Check sheet for the modelled part. Datum: model origin and axes. Units: mm. Round coordinates to 2 decimals unless told otherwise and drop trailing zeros. Loops run counter-clockwise (first coordinate to the right, second up) from the corner with the lowest first, then second, coordinate; pieces in that order, holes last. Notation, with made-up numbers: (48, 37.25) - (69, 37.25) arc R18 ccw to (69, 44.25) - close; hole circle Ø9 at (85, 34.25). An arc over 180 degrees is marked (long way). Put each result on its own line as item: value. Start each with the question number.
Item 1: Section check B-B, the plane x = 1.5. Record the cut outline in (y, z), and give its area (3 significant figures).
Item 2: Gauge pin test, flat ends, axial feed: pin 1 Ø4 at (x, y) = (5.5, -7.5) entering from -Z; pin 2 Ø2 at (x, z) = (3.5, -6) entering from +Y; pin 3 Ø6 at (x, z) = (7, -2) entering from -Y. Record the tip position at first contact, or that the pin passes through.
Item 3: Section check A-A, the plane y = 0. Record the cut outline in (x, z) (3 decimals).
Item 4: Draft check along Z on faces 1 (the flat face through (5.33, 7.76, 4.56)), 2 (the flat face through (5.33, 7.83, -4.44)), 3 (the cylindrical face through (5.33, -3.51, 3.82)), 4 (the flat face through (0, 2, -6)). Enter one of: pulls with the +Z half, pulls with the -Z half, needs draft (parallel to the pull), parting line crosses it, or undercut.
Item 5: Material ranges on line 1 along Z through (x, y) = (6.25, 0); line 2 along Z through (x, y) = (9.25, 3.75); line 3 along Y through (x, z) = (2, -1.75), recorded low to high.
Autodesk Inventor part; units mm, degrees
ref_plane "Work Plane1" through (-18.9656, 0, 0) normal (0, -0.8660254, -0.5) x (1, 0, 0)
ref_plane "YZ Plane" through (0, 0, 0) normal (1, 0, 0) x (0, 1, 0)
ref_plane "XZ Plane" through (0, 0, 0) normal (0, 1, 0) x (-1, 0, 0)
sketch "Эскиз1" plane through (0, 0, 0) normal (1, 0, 0) x (0, 1, 0)
  line L0 (-10.3923, 0) -> (-5.1962, 9)
  line L1 (-5.1962, 9) -> (5.1962, 9)
  line L2 (5.1962, 9) -> (10.3923, 0)
  line L3 (10.3923, 0) -> (5.1962, -9)
  line L4 (5.1962, -9) -> (-5.1962, -9)
  line L5 (-5.1962, -9) -> (-10.3923, 0)
  point P0 (0, 0)
  point P1 (0, 0)
  dimension "d0" = 20.7846
extrude "Базовый элемент" add sketch "Эскиз1" along normal blind 10.8
sketch "Эскиз2" plane through (0, 0, 0) normal (0, 0, 1) x (1, 0, 0)
  line L0 (0, 5.1962) -> (0, 10.3923)
  line L1 (0, 10.3923) -> (10.8, 10.3923)
  line L2 (10.8, 5.1962) -> (10.8, 10.3923)
  line L3 (-2.16, 0) -> (12.96, 0)
  line L4 (1.1993, 10.3923) -> (0, 8.315)
  line L5 (9.6007, 10.3923) -> (10.8, 8.315)
  dimension "d3" = 30
  dimension "d4" = 30
  dimension "d5" = 16.63
  dimension "d6" = 16.63
revolve "Фаска1" cut sketch "Эскиз2" angle 360 about axis through (-10, 0, 0) along (1, 0, 0)
sketch "Эскиз3" plane through (10.8, 0, 0) normal (1, 0, 0) x (0, 0, -1)
  arc A0 (-0.625, -1.0825) -> (0.625, -1.0825) centre (0, 0) ccw
hole "Резьба" at (10.8, 0, 0) direction (-1, 0, 0) diameter 10.376 end through all
chamfer "Фаска2" distance 0.8119 angle 30 1 edges at (10.8, 0, 5.188) measured on face at (10.8, 7.1795, -0.8718)
chamfer "Фаска3" distance 0.8119 angle 30 1 edges at (0, 0, 5.188) measured on face at (0, 7.1795, -0.8718)
ref_plane "Work Plane1" through (-18.9656, 0, 0) normal (0, -0.8660254, -0.5) x (1, 0, 0)
equation "\"d0\" = 1.1547 * SW"
equation "\"d1\" = KOH"
equation "\"d3\" = ANG1"
equation "\"d4\" = ANG2"
equation "\"d5\" = SW0"
equation "\"d6\" = SW01"
equation "\"d8\" = -0.5 * GD1 + 0.5 * NND"
equation "\"d40\" = -0.5 * GD1 + 0.5 * NND"
equation "\"d10\" = -0.5 * GD1 + 0.5 * NND"
equation "\"d41\" = -0.5 * GD1 + 0.5 * NND"
equation "\"ANG1\" = 30deg"
equation "\"ANG2\" = 30deg"
equation "\"NND\" = 12"
equation "\"KOH\" = 10.8"
equation "\"SW\" = 18"
equation "\"SW0\" = 16.63"
equation "\"SW01\" = SW0"
equation "\"GUL\" = 0.541266 * PTC"
equation "\"LADI\" = 12.345"
equation "\"TOA\" = 30deg"
equation "\"FAWI\" = 30deg"
equation "\"PTC\" = 1.5"
equation "\"THREADDIA\" = 12"
equation "\"E0\" = 1.155 * SW"
equation "\"GAL\" = 0.541266 * PTC"
properties part number "Копия гайки M12x1.5-6H ГОСТ 5915-70" material "Сталь, мягкая"
Check result:
1. outline: (-10.39, 0) - (-5.2, -9) - (5.2, -9) - (10.39, 0) - (5.2, 9) - (-5.2, 9) - close; hole circle Ø10.38 at (0, 0)
1. area: 196 mm²
2. pin 1: z = -8.47
2. pin 2: y = 7.51
2. pin 3: y = -10.39
3. outline: (0, -8.315) - (0.395, -9) - (10.405, -9) - (10.8, -8.315) - (10.8, -6) - (10.331, -5.188) - (0.469, -5.188) - (0, -6) - close; (0, 6) - (0.469, 5.188) - (10.331, 5.188) - (10.8, 6) - (10.8, 8.315) - (10.405, 9) - (0.395, 9) - (0, 8.315) - close
4. face 1: pulls with the +Z half
4. face 2: pulls with the -Z half
4. face 3: undercut
4. face 4: needs draft
5. line 1: -9 to -5.19, 5.19 to 9
5. line 2: -9 to -3.59, 3.59 to 9
5. line 3: -9.38 to -4.88, 4.88 to 9.38
